Can you work these out from the model? Positions are in its coordinate system, mm. A direction names the side the tool comes from. Round coordinates to 2 decimals unless told otherwise and drop trailing zeros. Order: outer loops, then holes, each group sorted by start corner. A loop starts at its lowest first (then second) coordinate and runs counter-clockwise, first axis right, second up. Notation, with made-up numbers: M -9.75,58.5 L 37.25,58.5 A17 ccw 37.25,68.5 Z; hole C 18.25,75 d6. An arc over 180 degrees is marked long. One line per question, with ' | ' between items.
Autodesk Inventor part; units mm, degrees
ref_plane "YZ Plane" through (0, 0, 0) normal (1, 0, 0) x (0, 1, 0)
ref_plane "XZ Plane" through (0, 0, 0) normal (0, 1, 0) x (-1, 0, 0)
ref_plane "XY Plane" through (0, 0, 0) normal (0, 0, 1) x (1, 0, 0)
sketch "Sketch1" plane through (0, 0, 0) normal (0, 0, 1) x (1, 0, 0)
  circle A0 centre (0, 0) radius 12.5
  circle A1 centre (0, 0) radius 4.5
  arc A2 (123.8397, -5) -> (123.8397, 5) centre (132.5, 0) ccw
  line L0 (11.4564, 5) -> (123.8397, 5)
  line L1 (12.5, -5) -> (123.8397, -5)
  line L2 (12.5, -5) -> (11.4564, -5)
  circle A3 centre (132.5, 0) radius 2.5
  dimension "d0" = 25
  dimension "d1" = 9
  dimension "d3" = 20
  dimension "d6" = 5
extrude "Extrusion1" add sketch "Sketch1" along normal blind 10 contours A0 | A0 L0 A2 L1 L2 | A1
extrude "Extrusion2" add sketch "Sketch1" against normal blind 5 contours A0
extrude "Extrusion3" add sketch "Sketch1" against normal blind 25 contours A1
properties part number "Rod" material "ABS Plastic"
(1) Will these pins go through, and if not, where does the flat tip stop? pin 1 Ø11 at (x, z) = (78.5, 5.5) entering from -Y; pin 2 Ø6 at (x, y) = (121.5, 4.5) entering from -Z; pin 3 Ø10 at (y, z) = (-10, 3) entering from -X.
Final values:
pin 1: y = -5 | pin 2: z = 0 | pin 3: x = -11.46
(2) If we section it at A-A on x = 132.5: Please give me the cut outline in (y, z).
Final values:
outline: M -10,0 L -2.5,0 L -2.5,10 L -10,10 Z; M 2.5,0 L 10,0 L 10,10 L 2.5,10 Z
(3) On a 3-axis mill with a long thin cutter (end or side, diameter ignored), from which of +Z, -Z, +X, -X, +Y, -Y can I reach the whole of each face in a straight line? I mean faces 1 (the flat face through (76, 0, 0)), 2 (the flat face through (0, 0, -25)), 3 (the flat face through (67, 5, 5)), 4 (the flat face through (0, -5, -5)), 5 (the cylindrical face through (134.885, -0.751, 4.93)). Say none if no direction works.
Final values:
face 1: -Z, +X, +Y, -Y | face 2: -Z, +X, -X, +Y, -Y | face 3: +Z, -Z, +Y | face 4: -Z | face 5: +Z, -Z
(4) If we section it at C-C on x = 0: Please give me the cut outline in (y, z).
Final values:
outline: M -12.5,-5 L -4.5,-5 L -4.5,-25 L 4.5,-25 L 4.5,-5 L 12.5,-5 L 12.5,10 L -12.5,10 Z
(5) If we section it at D-D on z = -22: Please give me the cut outline in (x, y).
Final values:
outline: C 0,0 d9
(6) Please list where these lines run through material, in increasing order: probe 1 along Y at (x, z) = (132.5, 5.25); probe 2 along Z at (x, y) = (1.5, 8.25); probe 3 along Y at (x, z) = (132, 6). Write a range as [from, to].
Final values:
probe 1: [-10, -2.5], [2.5, 10] | probe 2: [-5, 10] | probe 3: [-9.99, -2.45], [2.45, 9.99]
(7) Thinking about a two-plate mould opening in X: for faces 6 (the cylindrical face through (-0.59, 4.46, -14.86)), 7 (the flat face through (68, -5, 5)), 8 (the flat face through (64, 0, 10)), 9 (the cylindrical face through (142.493, 0.366, 4.93)), which applies, released by +X, released by -X, zero draft, split by the parting line, or undercut?
Final values:
face 6: split by the parting line | face 7: undercut | face 8: zero draft | face 9: undercut
(8) If we section it at B-B on y = 0: Please give me the cut outline in (x, z).
Final values:
outline: M -12.5,-5 L -4.5,-5 L -4.5,-25 L 4.5,-25 L 4.5,-5 L 12.5,-5 L 12.5,0 L 130,0 L 130,10 L -12.5,10 Z; M 135,0 L 142.5,0 L 142.5,10 L 135,10 Z
